from build123d import *

# Parameters (mm, degrees)
F2_R     = 4.8133
F3_DEPTH = 9.6012
F4_R     = 1.6002
F5_DEPTH = 22.1742


with BuildPart() as f1:
    # F0 (on Front) → F1 (revolve)
    with BuildSketch(Plane.XZ):
        with BuildLine():
            add(Edge.make_bspline(
                [(15.24, 13.4404166602), (24.9512382846, 17.761113573), (38.4288212127, 28.2685653314), (20.5129507573, 29.7235381078), (7.62, 31.2529022536)],
                knots=[0, 0, 0, 0, 0.4770419895, 1, 1, 1, 1], degree=3))
            Line((7.62, 31.2529022536), (7.62, 45.72))
            Line((7.62, 45.72), (0, 45.72))
            Line((0, 45.72), (0, 0))
            Line((0, 0), (15.24, 13.4404166602))
        make_face()
    revolve(axis=Axis((0, 0, 22.86), (0, 0, -1)))

    # F2 (on face) → F3 (cut)
    with BuildSketch(Plane.XY.offset(45.72)):
        Circle(F2_R)
    extrude(amount=-F3_DEPTH, mode=Mode.SUBTRACT)

    # F4 (on Top) → F5 (cut)
    with BuildSketch(Plane.XY):
        Circle(F4_R)
    extrude(amount=F5_DEPTH, mode=Mode.SUBTRACT)


solid = f1.part
Input: part model. Units: mm. Frame: model coordinates. A direction names the side the tool comes from. Give positions to 0.01 mm unless a question says otherwise; leave off trailing zeros. Loops run counter-clockwise (first coordinate to the right, second up) from the corner with the lowest first, then second, coordinate; pieces in that order, holes last. Notation, with made-up numbers: M 2.25,30.5 L 16.25,30.5 A29 cw 16.25,61.5 Z; hole C -26.5,-11.75 d9. An arc over 180 degrees is marked long. Use one line per item in the form item = value.
1. Pull-direction query (X, two-part tool) for faces 1 (the face through (-1.27, -0.974, 11.647)), 2 (the face through (3.786, -1.192, 3.5)), 3 (the face through (0, 0, 36.119)), 4 (the face through (0, 5, 45.72)); classes: released by +X, released by -X, zero draft, split by the parting line, or undercut.
Numbers:
face_1 = undercut
face_2 = split by the parting line
face_3 = undercut
face_4 = zero draft
2. Line query: L1, parallel to X at y = 0, z = 17; L2, parallel to Y at x = -1, z = 19.5; L3, parallel to Y at x = 0, z = 6.25. Output: solid intervals per line, ascending.
Numbers:
L1 = -22.25 to -1.6, 1.6 to 22.25
L2 = -26.06 to -1.25, 1.25 to 26.06
L3 = -7.09 to -1.6, 1.6 to 7.09
3. Section query A-A, the plane z = 37. Return the cut outline in (x, y), and give its area (3 significant figures).
Numbers:
outline = C 0,0 d15.24; hole C 0,0 d9.63
area = 110 mm²
4. Section query B-B, the plane z = 9. Return the cut outline in (x, y).
Numbers:
outline = C 0,0 d20.41; hole C 0,0 d3.2
5. Reachability of faces 5 (the face through (0, 0, 22.174)), 6 (the face through (-3.82, -2.93, 40.99)) from +Z, -Z, +X, -X, +Y, -Y: full face, straight path, thin tool, end or side. Return the list, or none.
Numbers:
face_5 = -Z
face_6 = +Z
6. First-contact query: pin 1 (1.5 mm diameter, centred on y = -21, z = 21.5, fed in from -X); pin 2 (5 mm diameter, centred on y = 18.5, z = 9.5, fed in from -X); pin 3 (1 mm diameter, centred on x = 0.5, y = -0.5, fed in from -Z); pin 4 (8 mm diameter, centred on x = 0.5, y = 15, fed in from +Z). Flat tips, straight axial feed; report the tip coordinate or a pass-through.
Numbers:
pin_1 = -20.55
pin_2 = through
pin_3 = 22.17
pin_4 = 30.86
